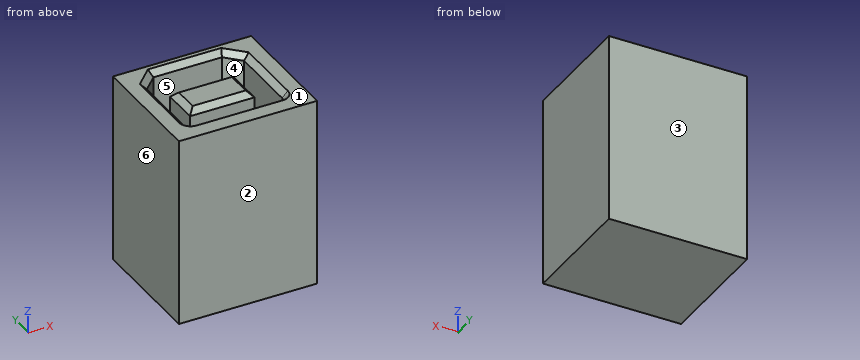
```python
from build123d import *

# Parameters (mm, degrees)
SKETCH_W        = 12
SKETCH_H        = 10.5
PAD_DEPTH       = 8.25
POCKET_DEPTH    = 9
SKETCH002_W     = 5.6
SKETCH002_H     = 3.18
PAD001_DEPTH    = 8.5
CHAMFER_SIZE    = 0.5
CHAMFER001_SIZE = 0.5


with BuildPart() as part:
    # Sketch → Pad (new body, symmetric)
    with BuildSketch(Plane.XY):
        Rectangle(SKETCH_W, SKETCH_H)
    extrude(amount=PAD_DEPTH, both=True)

    # Sketch001 → Pocket (cut)
    with BuildSketch(Plane.XY.offset(8.25)):
        with BuildLine():
            Line((-4.225, -2.93), (-4.225, 3.1))
            Line((-4.225, 3.1), (-2.975, 4.35))
            Line((-2.975, 4.35), (2.975, 4.35))
            Line((2.975, 4.35), (4.225, 3.1))
            Line((4.225, 3.1), (4.225, -2.93))
            ThreePointArc((3.725, -3.43), (4.078553, -3.283553), (4.225, -2.93))
            Line((3.725, -3.43), (-3.725, -3.43))
            ThreePointArc((-4.225, -2.93), (-4.078553, -3.283553), (-3.725, -3.43))
        make_face()
    extrude(amount=-POCKET_DEPTH, mode=Mode.SUBTRACT)

    # Sketch002 → Pad001 (new body)
    with BuildSketch(Plane.XY.offset(-0.75)):
        with Locations((0, 0.44)):
            Rectangle(SKETCH002_W, SKETCH002_H)
    extrude(amount=PAD001_DEPTH)

    # Chamfer
    chamfer_edges = [part.edges().sort_by_distance(p)[0] for p in [
        (2.8, 0.44, 7.75),
        (0, 2.03, 7.75),
        (-2.8, 0.44, 7.75),
        (0, -1.15, 7.75),
    ]]
    chamfer(chamfer_edges, length=CHAMFER_SIZE)

    # Chamfer001
    chamfer001_edges = [part.edges().sort_by_distance(p)[0] for p in [
        (0, -3.43, 8.25),
        (4.078553, -3.283553, 8.25),
        (-4.078553, -3.283553, 8.25),
        (4.225, 0.085, 8.25),
        (-4.225, 0.085, 8.25),
        (3.6, 3.725, 8.25),
        (-3.6, 3.725, 8.25),
        (0, 4.35, 8.25),
    ]]
    chamfer(chamfer001_edges, length=CHAMFER001_SIZE)


solid = part.part
```
Geometry check sheet. Reference: the model listing, model coordinates, mm. Face numbers are marked on the shaded views. A direction names the side the tool comes from. Round coordinates to 2 decimals unless told otherwise and drop trailing zeros. Order: outer loops, then holes, each group sorted by start corner. A loop starts at its lowest first (then second) coordinate and runs counter-clockwise, first axis right, second up. Notation, with made-up numbers: (77.5, -29.75) - (135.5, -29.75) arc R28 ccw to (135.5, -0.75) - close; hole circle Ø11 at (-17, 49). An arc over 180 degrees is marked (long way). Use a Markdown table: item, result. Add a question column.
(1) Release check for a two-part mould opening along Y. For the marked faces 1, 2, 3 and 4 record: pulls with the +Y half, pulls with the -Y half, needs draft (parallel to the pull), parting line crosses it, or undercut.
(2) Sectioned sample at D-D, the plane y = 0.75. Enter the section's corners in (x, z) (3 decimals), and give its area (3 significant figures).
(3) Material ranges on line 1 along Y through (x, z) = (-0.5, 6.75); line 2 along X through (y, z) = (-3, 2), recorded low to high. Write a range as [from, to].
(4) Tool access check on the marked faces 5 and 6. Record the directions out of +Z, -Z, +X, -X, +Y, -Y that give a thin tool (end or side, any length) a straight path to the whole face; none if there is none.
(5) Sectioned sample at A-A, the plane z = 3.25. Enter the section's corners in (x, y) (3 decimals), and give its area (3 significant figures).
(6) Sectioned sample at B-B, the plane y = 2.25. Enter the section's corners in (x, z) (3 decimals).
(7) Depth check by flat-ended pin: pin 1 (1.7 mm diameter, centred on x = -1, y = 1, fed in from +Z). Enter the tip coordinate at first touch or a pass-through.
(8) Sectioned sample at C-C, the plane x = 0.25. Enter the section's corners in (y, z).
Answers below:
| question | item | result |
|---|---|---|
| 1 | face 1 | needs draft |
| 1 | face 2 | pulls with the -Y half |
| 1 | face 3 | pulls with the +Y half |
| 1 | face 4 | undercut |
| 2 | outline | (-6, -8.25) - (6, -8.25) - (6, 8.25) - (4.725, 8.25) - (4.225, 7.75) - (4.225, -0.75) - (2.8, -0.75) - (2.8, 7.25) - (2.3, 7.75) - (-2.3, 7.75) - (-2.8, 7.25) - (-2.8, -0.75) - (-4.225, -0.75) - (-4.225, 7.75) - (-4.725, 8.25) - (-6, 8.25) - close |
| 2 | area | 169 mm² |
| 3 | line 1 | [-5.25, -3.43], [-1.15, 2.03], [4.35, 5.25] |
| 3 | line 2 | [-6, -4.22], [4.22, 6] |
| 4 | face 5 | +Z |
| 4 | face 6 | +Z, -Z, -X, +Y, -Y |
| 5 | outline | (-6, -5.25) - (6, -5.25) - (6, 5.25) - (-6, 5.25) - close; (-2.8, -1.15) - (2.8, -1.15) - (2.8, 2.03) - (-2.8, 2.03) - close; hole (-4.225, -2.93) arc R0.5 ccw to (-3.725, -3.43) - (3.725, -3.43) arc R0.5 ccw to (4.225, -2.93) - (4.225, 3.1) - (2.975, 4.35) - (-2.975, 4.35) - (-4.225, 3.1) - close |
| 5 | area | 79.7 mm² |
| 6 | outline | (-6, -8.25) - (6, -8.25) - (6, 8.25) - (4.725, 8.25) - (4.225, 7.75) - (4.225, -0.75) - (-4.225, -0.75) - (-4.225, 7.75) - (-4.725, 8.25) - (-6, 8.25) - close |
| 7 | pin 1 | z = 7.75 |
| 8 | outline | (-5.25, -8.25) - (5.25, -8.25) - (5.25, 8.25) - (4.85, 8.25) - (4.35, 7.75) - (4.35, -0.75) - (2.03, -0.75) - (2.03, 7.25) - (1.53, 7.75) - (-0.65, 7.75) - (-1.15, 7.25) - (-1.15, -0.75) - (-3.43, -0.75) - (-3.43, 7.75) - (-3.93, 8.25) - (-5.25, 8.25) - close |
